from build123d import *

# Parameters (mm, degrees)
BOSS_EXTRUDE1_DEPTH      = 2
BOSS_EXTRUDE2_DEPTH      = 17
SKETCH3_R                = 2.1
M4_CLEARANCE_HOLE1_D     = 4.8
M4_CLEARANCE_HOLE1_DEPTH = 2
M4_CLEARANCE_HOLE2_D     = 4.8
M4_CLEARANCE_HOLE2_DEPTH = 2


with BuildPart() as part:
    # Sketch1 → Boss-Extrude1 (new body)
    with BuildSketch(Plane(origin=(0, 0, 0), x_dir=(0, 0, -1), z_dir=(1, 0, 0))):
        Polygon((-38, 0), (0, 0), (0, 38), align=None)
    extrude(amount=BOSS_EXTRUDE1_DEPTH)

    # Sketch2 → Boss-Extrude2 (add)
    with BuildSketch(Plane(origin=(2, 0, 0), x_dir=(0, 0, -1), z_dir=(1, 0, 0))):
        Polygon((0, 38), (2, 38), (2, -2), (-38, -2), (-38, 0), (0, 0), align=None)
    extrude(amount=-BOSS_EXTRUDE2_DEPTH)

    # Sketch3 → Cut-Revolve1 (revolve, cut)
    with BuildSketch(Plane(origin=(0, 0, 0), x_dir=(1, 0, 0), z_dir=(0, 1, 0))):
        with Locations((-7.5, -10.089030863)):
            Circle(SKETCH3_R)
        with Locations((-7.5, -27.910969137)):
            Circle(SKETCH3_R)
    revolve(axis=Axis((-15, 0, 0), (1, 0, 0)), mode=Mode.SUBTRACT)

    # M4 Clearance Hole1
    with Locations(Plane.XY):
        with Locations((-7.5, 27.910969137), (-7.5, 10.089030863)):
            Hole(M4_CLEARANCE_HOLE1_D / 2, depth=M4_CLEARANCE_HOLE1_DEPTH)

    # M4 Clearance Hole2
    with Locations(Plane(origin=(0, 0, 0), x_dir=(1, 0, 0), z_dir=(0, 1, 0))):
        with Locations((-7.5, -10.089030863), (-7.5, -27.910969137)):
            Hole(M4_CLEARANCE_HOLE2_D / 2, depth=M4_CLEARANCE_HOLE2_DEPTH)


solid = part.part
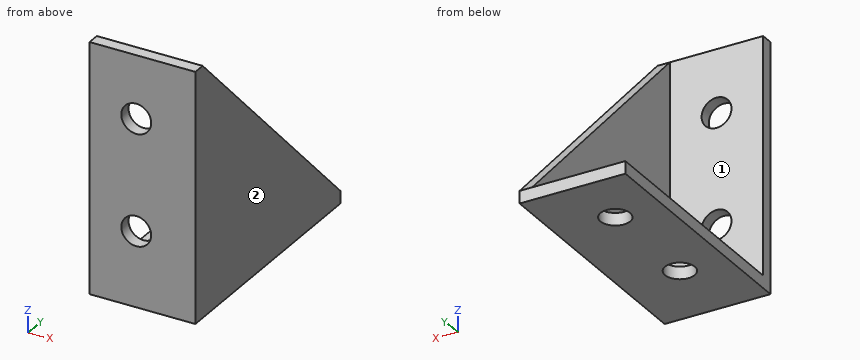
Could you check a few things on this model? Use its own coordinates, in mm. Face numbers are marked on the shaded views. A direction names the side the tool comes from. Give positions to 0.01 mm unless a question says otherwise; leave off trailing zeros. Write each loop counter-clockwise with the first axis right and the second up, starting at its lowest first coordinate (ties: lowest second). Pieces come first, ordered by that corner, then holes. Notation, with made-up numbers: (-7.75, -36.5) -> (29.25, -36.5) arc R23 cw to (29.25, -8.5) -> close; hole circle Ø4 at (35.5, 12). An arc over 180 degrees is marked (long way). Answer as CSV lines item,"result". Start each with the question number.
(1) If we section it at C-C, the plane z = 20: Write out the boundary of the cut face in (x, y), and give its area (3 significant figures).
(2) Which directions (+Z, -Z, +X, -X, +Y, -Y) give clear straight access to the entire face, cutting with the end or side of a thin tool? Please do the marked faces 1 and 2.
(3) I'm going to push flat-ended pins straight in: pin 1 Ø8 at (x, z) = (-11.5, 9.5) entering from +Y; pin 2 Ø4 at (y, z) = (8, 2.5) entering from -X; pin 3 Ø4 at (x, y) = (-7.5, 20.5) entering from +Z. Where does each tip first touch, or does it pass through?
(4) If we section it at D-D, the plane y = 9.5: Write out the boundary of the cut face in (x, z).
(5) If we section it at B-B, the plane y = 5: Write out the boundary of the cut face in (x, z).
(6) If we section it at A-A, the plane x = -7.5: Write out the boundary of the cut face in (y, z).
(7) Please list where these lines run through material, in increasing order: line 1 (Y direction, x = -7.5, z = -0.6); line 2 (Y direction, x = -4.5, z = 7.5).
Answer list:
1,outline,"(-15, -2) -> (2, -2) -> (2, 18) -> (0, 18) -> (0, 0) -> (-15, 0) -> close"
1,area,"70.0 mm^2"
2,face 1,"+Z, -X, +Y"
2,face 2,"+Z, -Z, +X, +Y, -Y"
3,pin 1,"y = 0"
3,pin 2,"x = 0"
3,pin 3,"z = 0"
4,outline,"(-15, -2) -> (-9.83, -2) -> (-9.83, 0) -> (-15, 0) -> close; (-5.17, -2) -> (2, -2) -> (2, 28.5) -> (0, 28.5) -> (0, 0) -> (-5.17, 0) -> close"
5,outline,"(-15, -2) -> (2, -2) -> (2, 33) -> (0, 33) -> (0, 0) -> (-15, 0) -> close"
6,outline,"(-2, -2) -> (7.69, -2) -> (7.69, 0) -> (0, 0) -> (0, 7.69) -> (-2, 7.69) -> close; (-2, 12.49) -> (0, 12.49) -> (0, 25.51) -> (-2, 25.51) -> close; (-2, 30.31) -> (0, 30.31) -> (0, 38) -> (-2, 38) -> close; (12.49, -2) -> (25.51, -2) -> (25.51, 0) -> (12.49, 0) -> close; (30.31, -2) -> (38, -2) -> (38, 0) -> (30.31, 0) -> close"
7,line 1,"-2 to 7.69, 12.49 to 25.51, 30.31 to 38"
7,line 2,"-2 to 0"
